Geometry: see drawing. Coordinates: mm, zero at the bounding-box minimum. Give positions to 0.01 mm unless a question says otherwise; leave off trailing zeros. Loops run counter-clockwise (first coordinate to the right, second up) from the corner with the lowest first, then second, coordinate; pieces in that order, holes last. Notation, with made-up numbers: M -2,16.5 L 6,16.5 A12 cw 6,21.5 Z; hole C -1,8.5 d6. An arc over 180 degrees is marked long. Put each result on its own line as item: value.
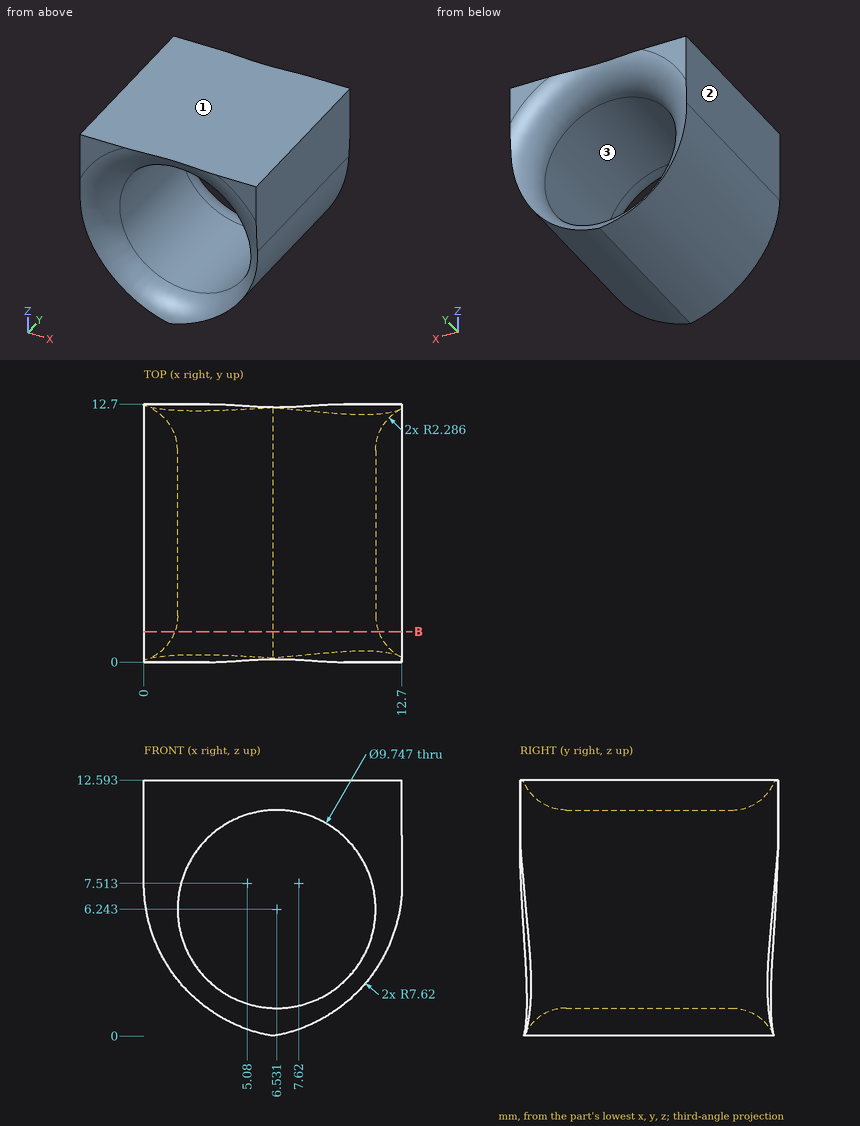
Item 1: Mould query, pull axis Z, two halves, no side actions, for the marked faces 1, 2 and 3. Classes: pulls with the +Z half, pulls with the -Z half, needs draft (parallel to the pull), parting line crosses it, or undercut.
Output values:
face 1: pulls with the +Z half
face 2: needs draft
face 3: undercut
Item 2: Pin query (flat end, axial travel): pin 1 Ø6 at (x, y) = (11, 9.5) entering from -Z (1 decimal); pin 2 Ø1 at (x, y) = (10.5, 7) entering from -Z (1 decimal); pin 3 Ø1 at (y, z) = (7, 6) entering from -X. Return the tip coordinate at first contact, or that it passes through.
Output values:
pin 1: z = 0.5
pin 2: z = 1.7
pin 3: x = 0.07
Item 3: Section B-B on y = 1.5. Output: boundary loops of the cut face in (x, z).
Output values:
outline: M 0,7.51 A7.62 ccw 6.35,0 A7.62 ccw 12.7,7.51 L 12.7,12.59 L 0,12.59 Z; hole C 6.53,6.24 d10.03
Item 4: Line query: probe 1 along Z at (x, y) = (6.5, 10.5); probe 2 along Z at (x, y) = (10.5, 1.5) (1 decimal); probe 3 along X at (y, z) = (5.75, 6.25) (1 decimal). Output: solid intervals per line, ascending. Write a range as [from, to].
Output values:
probe 1: [0.03, 1.37], [11.12, 12.59]
probe 2: [2.2, 3.2], [9.3, 12.6]
probe 3: [0.1, 1.7], [11.4, 12.6]
